Geometry check sheet. Reference: drawing and pictorial views, mm from the part's lowest x, y, z. A direction names the side the tool comes from. Round coordinates to 2 decimals unless told otherwise and drop trailing zeros. Write each loop counter-clockwise with the first axis right and the second up, starting at its lowest first coordinate (ties: lowest second). Pieces come first, ordered by that corner, then holes. Notation, with made-up numbers: (12, 55) - (36, 55) arc R23 ccw to (36, 86) - close; hole circle Ø4 at (65.5, 37). An arc over 180 degrees is marked (long way). Use one line per item in the form item = value. Start each with the question number.
1) Section check C-C (y = 10). Record the boundary of the cut face in (x, z), then the cut area to 3 significant figures.
2) Set-up check for the marked faces 1 and 2: record each of +Z, -Z, +X, -X, +Y, -Y from which the full face is reachable in a straight line by a thin tool's end or side.
3) Scan lines: probe 1 along X at (y, z) = (9.75, 35); probe 2 along X at (y, z) = (11.5, 15); probe 3 along Y at (x, z) = (7, 6). Record each from-to range of solid material in increasing order.
4) Draft check along X on the marked faces 3, 4, 5 and 6. Enter one of: +X half, -X half, draft (parallel to the pull), parting line (faces both ways), or undercut.
5) Section check A-A (z = 20). Record the boundary of the cut face in (x, y), then the cut area to 3 significant figures.
6) Gauge pin test, flat ends, axial feed: P1, Ø4, axis at x = 7, y = 10, coming from the -Z side; P2, Ø9, axis at x = 7, y = 10, coming from the +Z side. Record the tip position at first contact, or that the pin passes through.
7) Section check D-D (y = 13.75). Record the boundary of the cut face in (x, z), then the cut area to 3 significant figures.
8) Section check B-B (x = 20). Record the boundary of the cut face in (y, z), then the cut area to 3 significant figures.
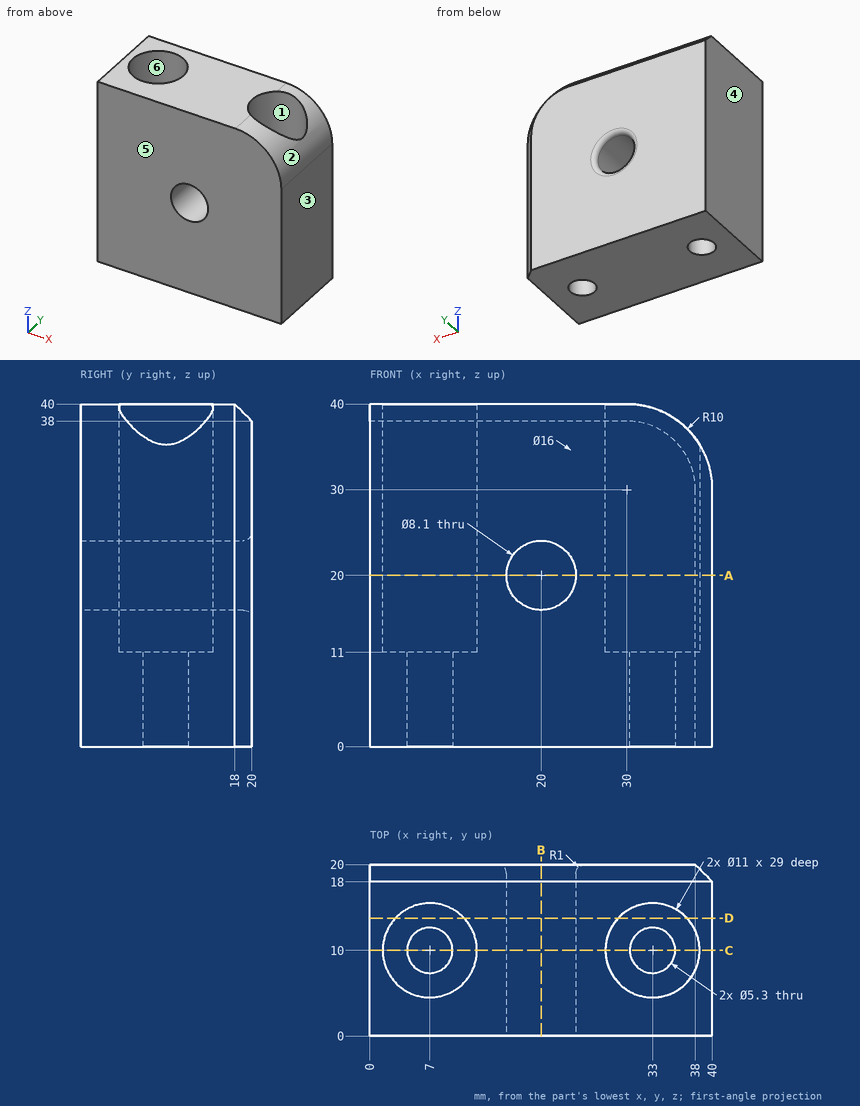
Results are:
q1.outline = (0, 0) - (4.35, 0) - (4.35, 11) - (1.5, 11) - (1.5, 40) - (0, 40) - close; (9.65, 0) - (30.35, 0) - (30.35, 11) - (27.5, 11) - (27.5, 40) - (12.5, 40) - (12.5, 11) - (9.65, 11) - close; (35.65, 0) - (40, 0) - (40, 30) arc R10 ccw to (38.5, 35.27) - (38.5, 11) - (35.65, 11) - close; hole circle Ø8.1 at (20, 20)
q1.area = 784 mm²
q2.face_1 = +Z
q2.face_2 = +Z, +X, +Y, -Y
q3.probe_1 = 0 to 1.51, 12.49 to 27.51, 38.49 to 38.66
q3.probe_2 = 0 to 1.71, 12.29 to 27.71, 38.29 to 40
q3.probe_3 = 0 to 7.35, 12.65 to 20
q4.face_3 = +X half
q4.face_4 = -X half
q4.face_5 = draft
q4.face_6 = undercut
q5.outline = (0, 0) - (15.95, 0) - (15.95, 19) arc R1 ccw to (14.95, 20) - (0, 20) - close; (24.05, 0) - (40, 0) - (40, 18) - (38, 20) - (25.05, 20) arc R1 ccw to (24.05, 19) - close; hole circle Ø11 at (7, 10); hole circle Ø11 at (33, 10)
q5.area = 446 mm²
q6.P1 = through
q6.P2 = 11
q7.outline = (0, 0) - (40, 0) - (40, 30) arc R10 ccw to (37.02, 37.12) - (37.02, 11) - (28.98, 11) - (28.98, 40) - (11.02, 40) - (11.02, 11) - (2.98, 11) - (2.98, 40) - (0, 40) - close; hole circle Ø8.1 at (20, 20)
q7.area = 1,070 mm²
q8.outline = (0, 0) - (20, 0) - (20, 14.95) arc R1 ccw to (19, 15.95) - (0, 15.95) - close; (0, 24.05) - (19, 24.05) arc R1 ccw to (20, 25.05) - (20, 38) - (18, 40) - (0, 40) - close
q8.area = 636 mm²
